```python
from build123d import *

# Parameters (mm, degrees)
SKETCH_1_R          = 25
SKETCH_1_R_2        = 17.35
EXTRUDE_1_DEPTH     = 100
SKETCH_2_W          = 150
SKETCH_2_H          = 163.350102445
SKETCH_2_W_2        = 100.72153761
SKETCH_2_H_2        = 448.495423617
CUT_EXTRUDE_1_DEPTH = 310
SKETCH_3_W          = 50
SKETCH_3_H          = 358.585755847
CUT_EXTRUDE_2_DEPTH = 310
FILLET_1_R          = 10


with BuildPart() as part:
    # 草图1 → 凸台-拉伸1 (new body, symmetric)
    with BuildSketch(Plane.XY):
        with BuildLine():
            Line((-94.612295013, 0), (-94.612295013, 410))
            ThreePointArc((-94.612295013, 410), (-49.57442783, 458.65476705), (2.407637637, 417.501872778))
            ThreePointArc((2.407637637, 417.501872778), (39.895934897, 220.789706501), (90.654933023, 27.07710262))
            ThreePointArc((90.654933023, 27.07710262), (13.682381008, -93.617727048), (-94.612295013, 0))
        make_face()
        Circle(SKETCH_1_R, mode=Mode.SUBTRACT)
        with Locations((-45.812295013, 410)):
            Circle(SKETCH_1_R_2, mode=Mode.SUBTRACT)
    extrude(amount=EXTRUDE_1_DEPTH, both=True)

    # 草图2 → 切除-拉伸1 (cut)
    with BuildSketch(Plane.ZY.offset(94.612295013)):
        with Locations((0, 421.675051222)):
            Rectangle(SKETCH_2_W, SKETCH_2_H)
        with Locations((-115.360768805, 85.752288191)):
            Rectangle(SKETCH_2_W_2, SKETCH_2_H_2)
        with Locations((115.360768805, 85.752288191)):
            Rectangle(SKETCH_2_W_2, SKETCH_2_H_2)
    extrude(amount=-CUT_EXTRUDE_1_DEPTH, mode=Mode.SUBTRACT)

    # 草图3 → 切除-拉伸2 (cut)
    with BuildSketch(Plane.ZY.offset(94.612295013)):
        with Locations((4.667160283, -95.292877924)):
            Rectangle(SKETCH_3_W, SKETCH_3_H)
    extrude(amount=-CUT_EXTRUDE_2_DEPTH, mode=Mode.SUBTRACT)

    # 圆角1
    fillet_1_edges = [part.edges().sort_by_distance(p)[0] for p in [
        (-39.543231053, 340, 75),
        (-39.543231053, 340, -75),
        (-36.717696937, 310, -100),
        (-36.717696937, 310, -65),
        (-36.717696937, 310, 100),
        (-36.717696937, 310, 65),
    ]]
    fillet(fillet_1_edges, radius=FILLET_1_R)


solid = part.part
```
Could you check a few things on this model? Use its own coordinates, in mm. A direction names the side the tool comes from. Round coordinates to 2 decimals unless told otherwise and drop trailing zeros. Loops run counter-clockwise (first coordinate to the right, second up) from the corner with the lowest first, then second, coordinate; pieces in that order, holes last.
Q1. I want a section at B-B (x = -8.5). Give the number of separate pieces and of enclosed holes in the cut face, and give its area (3 significant figures).
Q2. Thinking about a two-plate mould opening in Y: for faces 4 (the flat face through (-38, 310, 82)), 5 (the cylindrical face through (-37.806, 394.608, -87.675)), 6 (the cylindrical face through (39.279, 223.525, 1.4)), 7 (the cylindrical face through (-37.806, 394.608, 87.325)), which applies, pulls with the +Y half, pulls with the -Y half, needs draft (parallel to the pull), parting line crosses it, or undercut?
Q3. Please list where these lines run through material, in increasing order: L1, parallel to X at y = 0, z = 37; L2, parallel to Y at x = 0, z = -31; L3, parallel to Y at x = -49, z = 24.
Q4. On a 3-axis mill with a long thin cutter (end or side, diameter ignored), from which of +Z, -Z, +X, -X, +Y, -Y can I reach the whole of each face in a straight line? I mean faces 1 (the flat face through (-11, 84, 4)), 2 (the flat face through (-40, 340, -1)), 3 (the flat face through (-38, 310, -83)). Say none if no direction works.
Q5. For P1, Ø21, axis at x = -45.81, y = 410, coming from the +Z side (1 decimal); P2, Ø10, axis at x = 62.5, z = 2.5, coming from the -Y side; P3, Ø12, axis at x = -53.5, z = -84.5, coming from the -Y side; P4, Ø10, axis at x = 38, z = 66.5, coming from the -Y side, each with a flat end and sliding along its axis, tell me the tip position at first contact or that it passes through.
Q6. I want a section at A-A (y = 404). Write out the boundary of the cut face in (x, z).
Q7. I want a section at C-C (y = 72). Write out the boundary of the cut face in (x, z), and give its area (3 significant figures).
Q8. I want a section at D-D (z = 49). Write out the boundary of the cut face in (x, y), and give its area (3 significant figures).
Answer below:
1. separate pieces: 3
1. enclosed holes: 0
1. area: 51,000 mm2
2. face 4: pulls with the -Y half
2. face 5: undercut
2. face 6: pulls with the +Y half
2. face 7: undercut
3. L1: x = -94.61 to -25, 25 to 94.61
3. L2: y = -94.61 to -25, 25 to 340
3. L3: y = 84 to 340
4. face 1: +X, -X, -Y
4. face 2: +X, -X, +Y
4. face 3: -Z, +X, -X, -Y
5. P1: passes through
5. P2: stops at y = 84
5. P3: stops at y = 310
5. P4: stops at y = -88.58
6. outline: (-94.61, -100) - (-62.09, -100) - (-62.09, -75) - (-94.61, -75) - close; (-94.61, 75) - (-62.09, 75) - (-62.09, 100) - (-94.61, 100) - close; (-29.53, -100) - (4.54, -100) - (4.54, -75) - (-29.53, -75) - close; (-29.53, 75) - (4.54, 75) - (4.54, 100) - (-29.53, 100) - close
7. outline: (-94.61, -65) - (77.62, -65) - (77.62, -20.33) - (-94.61, -20.33) - close; (-94.61, 29.67) - (77.62, 29.67) - (77.62, 65) - (-94.61, 65) - close
7. area: 13,800 mm2
8. outline: (-94.61, 0) arc R94.61 ccw (long way) to (90.65, 27.08) arc R2947.42 cw to (15.53, 340) - (-94.61, 340) - close; hole circle Ø50 at (0, 0)
8. area: 62,500 mm2
